Design review of the part built by this model. Coordinates are the model's own, in mm. Face numbers are marked on the shaded views. A direction names the side the tool comes from. Give positions to 0.01 mm unless a question says otherwise; leave off trailing zeros. Loops run counter-clockwise (first coordinate to the right, second up) from the corner with the lowest first, then second, coordinate; pieces in that order, holes last. Notation, with made-up numbers: M -22,38.5 L 36,38.5 A22 cw 36,60.5 Z; hole C 29,48.25 d6. An arc over 180 degrees is marked long. Answer as CSV lines item,"result".
Autodesk Inventor part; units mm, degrees
ref_plane "YZ Plane" through (0, 0, 0) normal (1, 0, 0) x (0, 1, 0)
ref_plane "XZ Plane" through (0, 0, 0) normal (0, 1, 0) x (-1, 0, 0)
ref_plane "XY Plane" through (0, 0, 0) normal (0, 0, 1) x (1, 0, 0)
sketch "Sketch1" plane through (0, 0, 0) normal (0, 0, 1) x (1, 0, 0)
  line L0 (0, 0) -> (15, 0)
  line L1 (15, 0) -> (15, 10)
  line L2 (15, 10) -> (0, 10)
  line L3 (0, 10) -> (0, 0)
  line L4 (1, 9) -> (14, 9)
  line L5 (14, 9) -> (14, 1)
  line L6 (14, 1) -> (1, 1)
  line L7 (1, 1) -> (1, 9)
  dimension "d0" = 15
  dimension "d1" = 10
  dimension "d2" = 13
  dimension "d3" = 8
  dimension "d4" = 1
  dimension "d5" = 1
extrude "Extrusion1" add sketch "Sketch1" along normal blind 33
sketch "Sketch2" plane through (0, 10, 0) normal (0, 1, 0) x (1, 0, 0)
  line L0 (15, 0) -> (0, 0)
  line L1 (0, 0) -> (0, -33)
  line L2 (15, -33) -> (0, -33)
  line L3 (15, 0) -> (15, -33)
  circle A0 centre (5, -5) radius 1.5
  circle A1 centre (5, -28) radius 1.5
  dimension "d8" = 3
  dimension "d9" = 3
  dimension "d10" = 5
  dimension "d11" = 5
  dimension "d12" = 5
  dimension "d13" = 5
extrude "Extrusion2" cut sketch "Sketch2" against normal up to surface (10 mm away) contours A0 | A1
sketch "Sketch3" plane through (15, 0, 0) normal (1, 0, 0) x (0, 0, -1)
  line L0 (0, 0) -> (0, 10)
  line L1 (0, 10) -> (-33, 10)
  line L2 (-33, 0) -> (-33, 10)
  line L3 (0, 0) -> (-33, 0)
  circle A0 centre (-9, 5) radius 1.5
  circle A1 centre (-24, 5) radius 1.5
  dimension "d16" = 3
  dimension "d17" = 5
  dimension "d18" = 9
  dimension "d21" = 3
  dimension "d22" = 5
  dimension "d23" = 9
extrude "Extrusion3" cut sketch "Sketch3" against normal up to surface (15 mm away) contours A0 | A1
properties part number "profile2" material "Aluminum 6061, Welded"
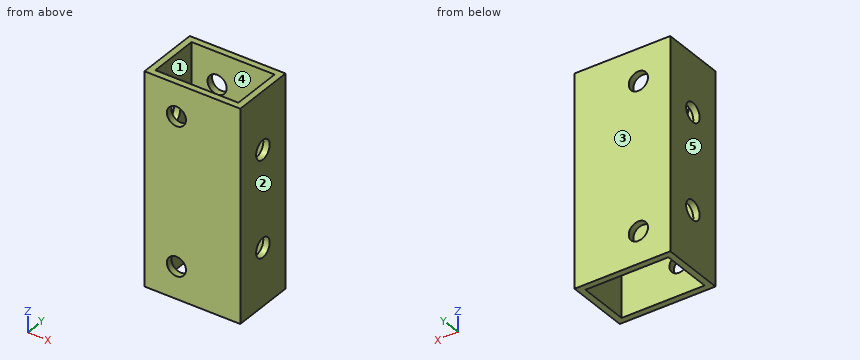
1. For P1, Ø2.5, axis at x = 5, z = 28, coming from the +Y side (1 decimal), flat-tipped, find the tip position at first contact; note if it passes through.
Answer block:
P1,"through"
2. For the marked faces 1 and 2, list the 3-axis set-ups (+Z, -Z, +X, -X, +Y, -Y) from which the entire face can be reached by the end or side of a thin tool; tool diameter is ignored.
Answer block:
face 1,"+Z, -Z"
face 2,"+Z, -Z, +X, +Y, -Y"
3. We need section A-A, the plane x = 5. Write out the cut boundary in (y, z).
Answer block:
outline,"M 0,0 L 1,0 L 1,3.5 L 0,3.5 Z; M 0,6.5 L 1,6.5 L 1,26.5 L 0,26.5 Z; M 0,29.5 L 1,29.5 L 1,33 L 0,33 Z; M 9,0 L 10,0 L 10,3.5 L 9,3.5 Z; M 9,6.5 L 10,6.5 L 10,26.5 L 9,26.5 Z; M 9,29.5 L 10,29.5 L 10,33 L 9,33 Z"
4. We need section B-B, the plane y = 5. Write out the cut boundary in (x, z).
Answer block:
outline,"M 0,0 L 1,0 L 1,7.5 L 0,7.5 Z; M 0,10.5 L 1,10.5 L 1,22.5 L 0,22.5 Z; M 0,25.5 L 1,25.5 L 1,33 L 0,33 Z; M 14,0 L 15,0 L 15,7.5 L 14,7.5 Z; M 14,10.5 L 15,10.5 L 15,22.5 L 14,22.5 Z; M 14,25.5 L 15,25.5 L 15,33 L 14,33 Z"
5. We need section D-D, the plane y = 7. Write out the cut boundary in (x, z).
Answer block:
outline,"M 0,0 L 1,0 L 1,33 L 0,33 Z; M 14,0 L 15,0 L 15,33 L 14,33 Z"
6. The part is to be moulded in two halves that separate along X. For the marked faces 3, 4 and 5, say which applies: pulls with the +X half, pulls with the -X half, needs draft (parallel to the pull), parting line crosses it, or undercut.
Answer block:
face 3,"needs draft"
face 4,"undercut"
face 5,"pulls with the -X half"
7. To check wall thickness, follow L1, parallel to X at y = 4.5, z = 10.5; L2, parallel to Z at x = 5, y = 0.4; L3, parallel to Y at x = 3, z = 22.5. State the ranges of each line that lie inside material, in increasing order. Write a range as [from, to].
Answer block:
L1,"[0, 1], [14, 15]"
L2,"[0, 3.5], [6.5, 26.5], [29.5, 33]"
L3,"[0, 1], [9, 10]"
8. We need section C-C, the plane z = 28. Write out the cut boundary in (x, y).
Answer block:
outline,"M 0,0 L 3.5,0 L 3.5,1 L 1,1 L 1,9 L 3.5,9 L 3.5,10 L 0,10 Z; M 6.5,0 L 15,0 L 15,10 L 6.5,10 L 6.5,9 L 14,9 L 14,1 L 6.5,1 Z"
